Autodesk Inventor part; units mm, degrees
ref_plane "YZ Plane" through (0, 0, 0) normal (1, 0, 0) x (0, 1, 0)
ref_plane "XZ Plane" through (0, 0, 0) normal (0, 1, 0) x (-1, 0, 0)
ref_plane "XY Plane" through (0, 0, 0) normal (0, 0, 1) x (1, 0, 0)
sketch "Sketch1" plane through (0, 0, 0) normal (0, 0, 1) x (1, 0, 0)
  line L0 (3, 0) -> (3, -15)
  line L1 (3, -15) -> (1, -15)
  line L2 (1, -15) -> (1, -2)
  line L3 (1, -2) -> (-12, -2)
  line L4 (-12, -2) -> (-12, 0)
  line L5 (-12, 0) -> (3, 0)
  line L6 (-12, 0) -> (3, 0)
  dimension "d38" = 2
  dimension "d39" = 13
  dimension "d40" = 13
  dimension "d41" = 2
extrude "Extrusion3" add sketch "Sketch1" along normal blind 15
sketch "Sketch2" plane through (-12, -2, 0) normal (0, -1, 0) x (1, 0, 0)
  circle A0 centre (4, 3.5) radius 1.5
  line L0 (0, 15) -> (13, 15)
  line L1 (0, 0) -> (0, 15)
  line L2 (0, 0) -> (13, 0)
  circle A1 centre (4, 11.5) radius 1.5
  dimension "d45" = 3
  dimension "d47" = 4
  dimension "d48" = 3.5
  dimension "d49" = 3
  dimension "d50" = 4
  dimension "d51" = 3.5
extrude "Extrusion4" cut sketch "Sketch2" against normal blind 10
sketch "Sketch3" plane through (1, -15, 0) normal (-1, 0, 0) x (0, 0, 1)
  circle A0 centre (10.75, 5.375) radius 1
  circle A1 centre (4.25, 5.375) radius 1
  line L0 (0, 0) -> (15, 0)
  line L1 (15, 13) -> (15, 0)
  line L2 (0, 13) -> (0, 0)
  circle A2 centre (7.5, 10) radius 2
  dimension "d54" = 2
  dimension "d55" = 2
  dimension "d56" = 5.375
  dimension "d57" = 5.375
  dimension "d58" = 4.25
  dimension "d59" = 4.25
  dimension "d62" = 4
  dimension "d65" = 10
extrude "Extrusion5" cut sketch "Sketch3" against normal blind 10 contours A0 | A1
extrude "Extrusion6" cut sketch "Sketch3" against normal blind 10 contours A2
fillet "Fillet1" radius 2.5 1 edges at (3, 0, 7.5)
fillet "Fillet2" radius 0.5 1 edges at (1, -2, 7.5)
equation "\"d51\" = d48"
equation "\"d58\" = d59"
properties part number "Soporte de Final de Carrera - Eje X" material "Aluminum 1100-H14"
Work out the finished part from the listing and answer in its coordinate system (mm). A direction names the side the tool comes from. Give positions to 0.01 mm unless a question says otherwise; leave off trailing zeros. Order: outer loops, then holes, each group sorted by start corner. A loop starts at its lowest first (then second) coordinate and runs counter-clockwise, first axis right, second up. Notation, with made-up numbers: M 45.25,86.25 L 70.25,86.25 A33 cw 70.25,118.25 Z; hole C 28.25,-5 d4. An arc over 180 degrees is marked long. Return JSON: item names as keys, results as strings.
1) Section A-A, the plane z = 7.5 is taken. Write down the section's boundary in (x, y).
Resolved:
{"outline": "M -12,-2 L 0.5,-2 A0.5 cw 1,-2.5 L 1,-3 L 3,-3 L 3,-2.5 A2.5 ccw 0.5,0 L -12,0 Z; M 1,-15 L 3,-15 L 3,-7 L 1,-7 Z"}
2) Each of these flat-tipped pins is pushed along its axis until it touches: pin 1 (3 mm diameter, centred on x = -8.5, z = 4, fed in from -Y); pin 2 (6 mm diameter, centred on y = -8.5, z = 2, fed in from -X). Where does it stop, or does it pass through?
Resolved:
{"pin 1": "y = -2", "pin 2": "x = 1"}
3) A tool of negligible diameter and unlimited length cuts with its end or side. For faces 4 (the flat face through (-6, -2, 7)), 5 (the cylindrical face through (-9.5, -1.01, 11.57)), from which of +Z, -Z, +X, -X, +Y, -Y can it reach the whole face along a straight path? Write none if from no direction.
Resolved:
{"face 4": "+Z, -Z, -X, -Y", "face 5": "+Y, -Y"}
4) Section C-C, the plane x = -9.25 is taken. Write down the section's boundary in (y, z), plus the area to 3 significant figures.
Resolved:
{"outline": "M -2,0 L 0,0 L 0,2.67 L -2,2.67 Z; M -2,4.33 L 0,4.33 L 0,10.67 L -2,10.67 Z; M -2,12.33 L 0,12.33 L 0,15 L -2,15 Z", "area": "23.4 mm^2"}
5) Section B-B, the plane z = 10.75 is taken. Write down the section's boundary in (x, y) (3 decimals).
Resolved:
{"outline": "M -12,-2 L -9.299,-2 L -9.299,0 L -12,0 Z; M -6.701,-2 L 0.5,-2 A0.5 cw 1,-2.5 L 1,-8.625 L 3,-8.625 L 3,-2.5 A2.5 ccw 0.5,0 L -6.701,0 Z; M 1,-15 L 3,-15 L 3,-10.625 L 1,-10.625 Z"}
6) Section D-D, the plane y = -4 is taken. Write down the section's boundary in (x, z).
Resolved:
{"outline": "M 1,0 L 3,0 L 3,5.77 L 1,5.77 Z; M 1,9.23 L 3,9.23 L 3,15 L 1,15 Z"}
7) For a pull along Y with two mould halves and no side action, classify faces 1 (the flat face through (1, -9, 7)), 2 (the cylindrical face through (2.287, -0.752, 7.605)), 3 (the cylindrical face through (1.986, -8.634, 10.62)) as +Y half, -Y half, draft (parallel to the pull), parting line (faces both ways), or undercut.
Resolved:
{"face 1": "draft", "face 2": "+Y half", "face 3": "undercut"}
8) Straight lines are drawn through the part: line 1 along Z through (x, y) = (-8, -0.5); line 2 along X through (y, z) = (-8.5, 13); line 3 along Y through (x, z) = (2.4, 10.75) (3 decimals). For each, find the intervals that lie inside material, in ascending order. Write a range as [from, to].
Resolved:
{"line 1": "[0, 2], [5, 10], [13, 15]", "line 2": "[1, 3]", "line 3": "[-15, -10.625], [-8.625, -0.875]"}
